For this review, use the dimensioned drawing (mm, ordinates from the lowest corner) and the shaded views. A direction names the side the tool comes from. Coordinates: 2 decimals unless noted, no trailing zeros. Write each loop counter-clockwise with the first axis right and the second up, starting at its lowest first coordinate (ties: lowest second). Pieces come first, ordered by that corner, then holes. Notation, with made-up numbers: (9, -32) - (54, -32) arc R12 cw to (54, -26) - close; hole circle Ø10 at (-32, 11.5). An arc over 180 degrees is marked (long way). Answer as a JSON object with one key per item and string values.
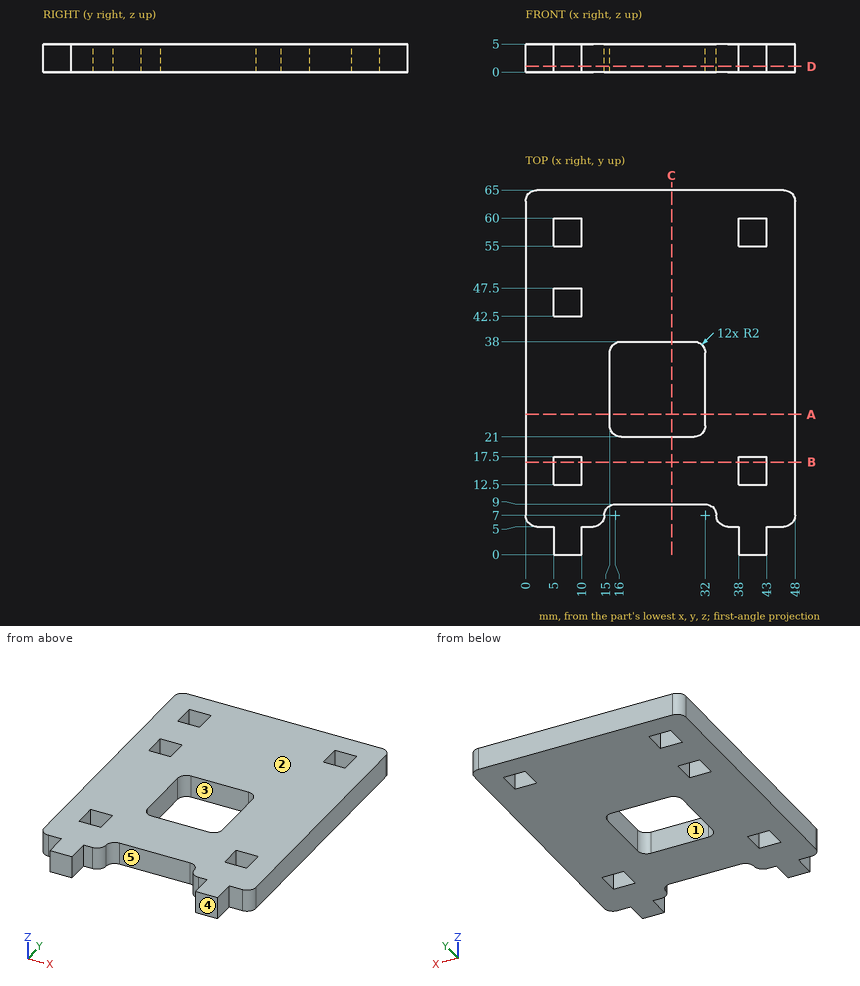
(1) Take a section at A-A, the plane y = 25. Write out the cut boundary in (x, z), and give its area (3 significant figures).
Solved:
{"outline": "(0, 0) - (15, 0) - (15, 5) - (0, 5) - close; (32, 0) - (48, 0) - (48, 5) - (32, 5) - close", "area": "155 mm^2"}
(2) To check wall thickness, follow line 1 (Y direction, x = 39, z = 3.35); line 2 (Y direction, x = 7, z = 3.95); line 3 (X direction, y = 15, z = 2.35). State the ranges of each line that lie inside material, in increasing order. Write a range as from..to.
Solved:
{"line 1": "y = 0..12.5, 17.5..55, 60..65", "line 2": "y = 0..12.5, 17.5..42.5, 47.5..55, 60..65", "line 3": "x = 0..5, 10..38, 43..48"}
(3) Take a section at D-D, the plane z = 1. Give the number of separate pieces and of enclosed holes in the cut face, and give its area (3 significant figures).
Solved:
{"separate pieces": "1", "enclosed holes": "6", "area": "2,440 mm^2"}
(4) Tool access review of the marked faces 4 and 5: name each direction out of +Z, -Z, +X, -X, +Y, -Y from which nothing blocks a thin tool from reaching the whole face with its end or side.
Solved:
{"face 4": "+Z, -Z, +X, -X, -Y", "face 5": "+Z, -Z, -Y"}
(5) Take a section at C-C, the plane x = 26. Write out the cut boundary in (y, z).
Solved:
{"outline": "(9, 0) - (21, 0) - (21, 5) - (9, 5) - close; (38, 0) - (65, 0) - (65, 5) - (38, 5) - close"}
(6) The part is to be moulded in two halves that separate along X. For the marked faces 1, 2 and 3, say which applies: pulls with the +X half, pulls with the -X half, needs draft (parallel to the pull), parting line crosses it, or undercut.
Solved:
{"face 1": "undercut", "face 2": "needs draft", "face 3": "undercut"}
(7) For pin 1 (2.5 mm diameter, centred on x = 25.5, z = 2, fed in from -Y); pin 2 (1.5 mm diameter, centred on y = 3.5, z = 2, fed in from +X), all flat-tipped, find the tip position at first contact; note any pin that passes through.
Solved:
{"pin 1": "stops at y = 9", "pin 2": "stops at x = 43"}
(8) Take a section at B-B, the plane y = 16.5. Write out the cut boundary in (x, z).
Solved:
{"outline": "(0, 0) - (5, 0) - (5, 5) - (0, 5) - close; (10, 0) - (38, 0) - (38, 5) - (10, 5) - close; (43, 0) - (48, 0) - (48, 5) - (43, 5) - close"}
